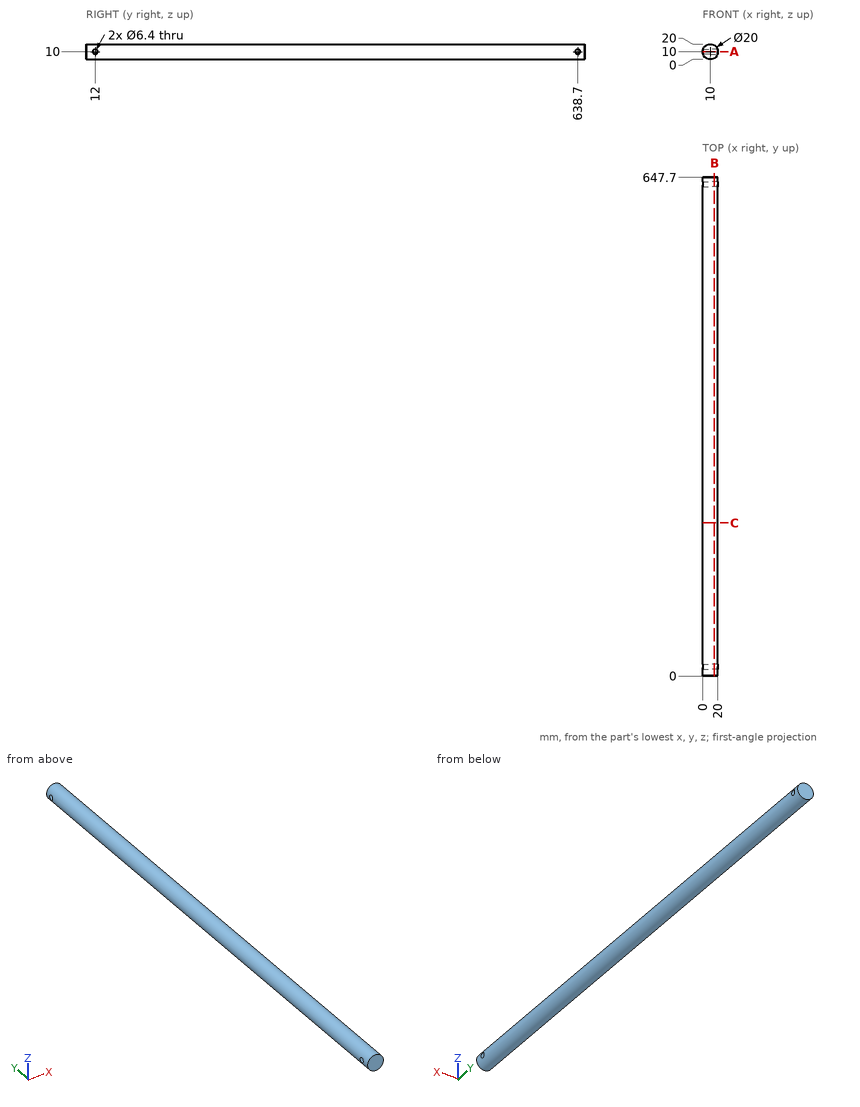
Verification items for this drawing (mm, ordinates from the low corner). Give positions to 0.01 mm unless a question says otherwise; leave off trailing zeros. Loops run counter-clockwise (first coordinate to the right, second up) from the corner with the lowest first, then second, coordinate; pieces in that order, holes last. Notation, with made-up numbers: M 32,57.5 L 61,57.5 A15 cw 61,86.5 Z; hole C 87,-29 d6. An arc over 180 degrees is marked long. Write item = value, one per line.
(1) Material ranges on line 1 (Y direction, x = 15.5, z = 10.75); line 2 (Y direction, x = 6.25, z = 10); line 3 (Z direction, x = 9.5, y = 268), recorded low to high. Write a range as [from, to].
Answer below:
line_1 = [0, 8.89], [15.11, 635.59], [641.81, 647.7]
line_2 = [0, 8.8], [15.2, 635.5], [641.9, 647.7]
line_3 = [0.01, 19.99]
(2) Sectioned sample at A-A, the plane z = 10. Record the cut outline in (x, y), plus the area to 3 significant figures.
Answer below:
outline = M 0,0 L 20,0 L 20,8.8 L 0,8.8 Z; M 0,15.2 L 20,15.2 L 20,635.5 L 0,635.5 Z; M 0,641.9 L 20,641.9 L 20,647.7 L 0,647.7 Z
area = 12,700 mm2
(3) Gauge pin test, flat ends, axial feed: pin 1 Ø5 at (x, y) = (14.5, 101) entering from -Z; pin 2 Ø6 at (y, z) = (525.5, 13.5) entering from +X; pin 3 Ø4 at (y, z) = (638.7, 10) entering from +X; pin 4 Ø5 at (x, y) = (4, 186) entering from +Z. Record the tip position at first contact, or that the pin passes through.
Answer below:
pin_1 = 0.2
pin_2 = 19.99
pin_3 = through
pin_4 = 19.37
(4) Sectioned sample at C-C, the plane y = 199. Record the cut outline in (x, z), plus the area to 3 significant figures.
Answer below:
outline = C 10,10 d20
area = 314 mm2
(5) Sectioned sample at B-B, the plane x = 15.25. Record the cut outline in (y, z).
Answer below:
outline = M 0,1.49 L 647.7,1.49 L 647.7,18.51 L 0,18.51 Z; hole C 12,10 d6.4; hole C 638.7,10 d6.4
